from build123d import *

# Parameters (mm, degrees)
SKETCH_1_R      = 3.5
SKETCH_1_R_2    = 0.95
EXTRUDE_2_DEPTH = 1.5


with BuildPart() as part:
    # 草图1 → 凸台-拉伸2 (new body)
    with BuildSketch(Plane.XY):
        with BuildLine():
            ThreePointArc((-5, 4.898979486), (0, -7), (5, 4.898979486))
            Line((5, 4.898979486), (5, 40.25))
            Line((5, 40.25), (-5, 40.25))
            Line((-5, 40.25), (-5, 4.898979486))
        make_face()
        Circle(SKETCH_1_R, mode=Mode.SUBTRACT)
        with Locations((0, 36.25)):
            Circle(SKETCH_1_R_2, mode=Mode.SUBTRACT)
        with Locations((0, 9.95)):
            Circle(SKETCH_1_R_2, mode=Mode.SUBTRACT)
        with Locations((0, 12.85)):
            Circle(SKETCH_1_R_2, mode=Mode.SUBTRACT)
        with Locations((0, 15.75)):
            Circle(SKETCH_1_R_2, mode=Mode.SUBTRACT)
        with Locations((0, 29.35)):
            Circle(SKETCH_1_R_2, mode=Mode.SUBTRACT)
    extrude(amount=EXTRUDE_2_DEPTH)


solid = part.part
Verification items for the finished model (mm, model axes). A direction names the side the tool comes from. Give positions to 0.01 mm unless a question says otherwise; leave off trailing zeros. Write each loop counter-clockwise with the first axis right and the second up, starting at its lowest first coordinate (ties: lowest second). Pieces come first, ordered by that corner, then holes. Notation, with made-up numbers: (65, 51.5) - (103, 51.5) arc R18 cw to (103, 69.5) - close; hole circle Ø2 at (77.25, 29). An arc over 180 degrees is marked (long way). Answer as CSV lines item,"result". Start each with the question number.
1. Sectioned sample at C-C (x = -2). Record the boundary of the cut face in (y, z), then the cut area to 3 significant figures.
2. Sectioned sample at B-B (y = 0). Record the boundary of the cut face in (x, z), then the cut area to 3 significant figures.
3. Set-up check for faces 1 (the face through (5, 22, 1)), 2 (the face through (-0.206, 35.323, 0.74)), 3 (the face through (-5, 23, 1)): record each of +Z, -Z, +X, -X, +Y, -Y from which the full face is reachable in a straight line by a thin tool's end or side.
4. Sectioned sample at D-D (z = 0.25). Record the boundary of the cut face in (x, y), then the cut area to 3 significant figures.
5. Draft check along Y on faces 4 (the face through (-0.124, 30.292, 0.74)), 5 (the face through (0, -7, 1)), 6 (the face through (0, 17, 0)). Enter one of: pulls with the +Y half, pulls with the -Y half, needs draft (parallel to the pull), parting line crosses it, or undercut.
6. Thickness scan on line 1 (X direction, y = 32, z = 0.2); line 2 (Y direction, x = -1, z = 0.95); line 3 (X direction, y = 2.5, z = 0.15). Record the ranges inside material, lowest first.
7. Sectioned sample at A-A (x = 0). Record the boundary of the cut face in (y, z).
8. Depth check by flat-ended pin: pin 1 (2 mm diameter, centred on x = 0, y = 29.35, fed in from +Z). Enter the tip coordinate at first touch or a pass-through.
Derived:
1,outline,"(-6.71, 0) - (-2.87, 0) - (-2.87, 1.5) - (-6.71, 1.5) - close; (2.87, 0) - (40.25, 0) - (40.25, 1.5) - (2.87, 1.5) - close"
1,area,"61.8 mm²"
2,outline,"(-7, 0) - (-3.5, 0) - (-3.5, 1.5) - (-7, 1.5) - close; (3.5, 0) - (7, 0) - (7, 1.5) - (3.5, 1.5) - close"
2,area,"10.5 mm²"
3,face 1,"+Z, -Z, +X, +Y"
3,face 2,"+Z, -Z"
3,face 3,"+Z, -Z, -X, +Y"
4,outline,"(-5, 4.9) arc R7 ccw (long way) to (5, 4.9) - (5, 40.25) - (-5, 40.25) - close; hole circle Ø7 at (0, 0); hole circle Ø1.9 at (0, 9.95); hole circle Ø1.9 at (0, 12.85); hole circle Ø1.9 at (0, 15.75); hole circle Ø1.9 at (0, 29.35); hole circle Ø1.9 at (0, 36.25)"
4,area,"440 mm²"
5,face 4,"undercut"
5,face 5,"parting line crosses it"
5,face 6,"needs draft"
6,line 1,"-5 to 5"
6,line 2,"-6.93 to -3.35, 3.35 to 40.25"
6,line 3,"-6.54 to -2.45, 2.45 to 6.54"
7,outline,"(-7, 0) - (-3.5, 0) - (-3.5, 1.5) - (-7, 1.5) - close; (3.5, 0) - (9, 0) - (9, 1.5) - (3.5, 1.5) - close; (10.9, 0) - (11.9, 0) - (11.9, 1.5) - (10.9, 1.5) - close; (13.8, 0) - (14.8, 0) - (14.8, 1.5) - (13.8, 1.5) - close; (16.7, 0) - (28.4, 0) - (28.4, 1.5) - (16.7, 1.5) - close; (30.3, 0) - (35.3, 0) - (35.3, 1.5) - (30.3, 1.5) - close; (37.2, 0) - (40.25, 0) - (40.25, 1.5) - (37.2, 1.5) - close"
8,pin 1,"z = 1.5"
